```python
from build123d import *

# Parameters (mm, degrees)
F0_W     = 203.2
F0_H     = 241.3
F1_DEPTH = 9.525
F2_W     = 28.575
F2_H     = 9.525
F3_DEPTH = 4.7625
F4_W     = 28.575
F4_H     = 9.525
F5_DEPTH = 3.175
F6_R     = 3.17499


# Not quite as in the source:
# - a fillet or chamfer is up to 0.001 mm smaller than in the source, because OpenCascade refuses the exact size


with BuildPart() as f1:
    # F0 (on Top) → F1 (new body)
    with BuildSketch(Plane.XY):
        Rectangle(F0_W, F0_H)
    extrude(amount=F1_DEPTH)

    # F2 (on face) → F3 (cut)
    with BuildSketch(Plane.XZ.offset(120.65)):
        with Locations((15.875, 4.7625)):
            Rectangle(F2_W, F2_H)
    extrude(amount=-F3_DEPTH, mode=Mode.SUBTRACT)

    # F4 (on face) → F5 (cut)
    with BuildSketch(Plane(origin=(0, 120.65, 0), x_dir=(-1, 0, 0), z_dir=(0, 1, 0))):
        with Locations((-41.275, 4.7625)):
            Rectangle(F4_W, F4_H)
        with Locations((9.525, 4.7625)):
            Rectangle(F4_W, F4_H)
    extrude(amount=-F5_DEPTH, mode=Mode.SUBTRACT)

    # F6 (radius 3.175 in the source; OpenCascade refuses exactly that, so slightly less here)
    f6_edges = [f1.edges().sort_by_distance(p)[0] for p in [
        (-101.6, 120.65, 4.7625),
        (-23.8125, 120.65, 4.7625),
        (4.7625, 120.65, 4.7625),
        (26.9875, 120.65, 4.7625),
        (55.5625, 120.65, 4.7625),
        (101.6, 120.65, 4.7625),
        (-101.6, -120.65, 4.7625),
        (1.5875, -120.65, 4.7625),
        (30.1625, -120.65, 4.7625),
        (101.6, -120.65, 4.7625),
    ]]
    fillet(f6_edges, radius=F6_R)


solid = f1.part
```
Source: CAD feature listing. Evaluate the final solid. Frame: model axes, mm. A direction names the side the tool comes from. Give positions to 0.01 mm unless a question says otherwise; leave off trailing zeros. Use CSV: the item, a comma, the result in double quotes. Start each with the question number.
1. Draft query along X for faces 3 (the flat face through (41, 117.475, 5)), 4 (the flat face through (16, -115.888, 5)), 5 (the flat face through (-101.6, -2, 5)), 6 (the flat face through (16, 120.65, 5)). Return one class per face: +X half, -X half, draft (parallel to the pull), parting line (faces both ways), or undercut.
2. Pin query (flat end, axial travel): pin 1 (4 mm diameter, centred on x = 52.5, z = 4.5, fed in from +Y) (3 decimals); pin 2 (5 mm diameter, centred on x = 21.5, z = 4.5, fed in from -Y). Return the tip coordinate at first contact, or that it passes through.
3. Ray query, L1, parallel to Y at x = 15, z = 3; L2, parallel to Y at x = 28.5, z = 9 (1 decimal). Return the intervals inside material, ascending.
4. Reachability of faces 1 (the flat face through (-9, 117.475, 5)), 2 (the flat face through (-1, 2, 9.525)) from +Z, -Z, +X, -X, +Y, -Y: full face, straight path, thin tool, end or side. Return the list, or none.
Response:
1,face 3,"undercut"
1,face 4,"undercut"
1,face 5,"-X half"
1,face 6,"draft"
2,pin 1,"y = 117.475"
2,pin 2,"y = -115.89"
3,L1,"-115.89 to 120.65"
3,L2,"-115.9 to 117.5"
4,face 1,"+Z, -Z, +Y"
4,face 2,"+Z, +X, -X, +Y, -Y"
